from build123d import *

# Parameters (mm, degrees)
F1_DEPTH = 50.8
F2_W     = 25.4
F2_H     = 15.875
F3_DEPTH = 19.05


with BuildPart() as f1:
    # F0 (on Right) → F1 (new body)
    with BuildSketch(Plane.YZ):
        with BuildLine():
            Line((0, 0), (0, 38.1))
            Line((0, 38.1), (-6.35, 38.1))
            ThreePointArc((-6.35, 38.1), (-10.069744, 16.419744), (-31.75, 12.7))
            Line((-31.75, 12.7), (-31.75, 0))
            Line((-31.75, 0), (0, 0))
        make_face()
    extrude(amount=F1_DEPTH)

    # F2 (on face) → F3 (cut)
    with BuildSketch(Plane.XY.offset(38.1)):
        with Locations((25.4, -7.9375)):
            Rectangle(F2_W, F2_H)
    extrude(amount=-F3_DEPTH, mode=Mode.SUBTRACT)


solid = f1.part
Verification items for the finished model (mm, model axes). A direction names the side the tool comes from. Give positions to 0.01 mm unless a question says otherwise; leave off trailing zeros. Write each loop counter-clockwise with the first axis right and the second up, starting at its lowest first coordinate (ties: lowest second). Pieces come first, ordered by that corner, then holes. Notation, with made-up numbers: (-17, 69) - (5, 69) arc R24 ccw to (5, 108) - close; hole circle Ø8 at (83.25, -12). An arc over 180 degrees is marked (long way). Answer as CSV lines item,"result". Start each with the question number.
1. Sectioned sample at B-B (x = 6). Record the boundary of the cut face in (y, z), then the cut area to 3 significant figures.
2. Draft check along X on faces 3 (the face through (12.7, -3, 29)), 4 (the face through (44, -3, 38.1)), 5 (the face through (50.8, -13, 11)), 6 (the face through (0, -13, 11)). Enter one of: pulls with the +X half, pulls with the -X half, needs draft (parallel to the pull), parting line crosses it, or undercut.
3. Sectioned sample at D-D (z = 22). Record the boundary of the cut face in (x, y).
4. Depth check by flat-ended pin: pin 1 (4 mm diameter, centred on x = 7, z = 20, fed in from -Y); pin 2 (12 mm diameter, centred on x = 33.5, y = -25, fed in from +Z); pin 3 (12 mm diameter, centred on y = -26, z = 23, fed in from -X); pin 4 (2.5 mm diameter, centred on x = 26.5, y = -5.5, fed in from +Z). Enter the tip coordinate at first touch or a pass-through.
5. Thickness scan on line 1 (X direction, y = -1.5, z = 20.5); line 2 (Z direction, x = 20.5, y = -7.5); line 3 (Z direction, x = 24, y = -24). Record the ranges inside material, lowest first.
6. Sectioned sample at A-A (z = 35.5). Record the boundary of the cut face in (x, y), then the cut area to 3 significant figures.
7. Sectioned sample at C-C (y = -5.5). Record the boundary of the cut face in (x, z).
8. Set-up check for faces 1 (the face through (38.1, -3, 29)), 2 (the face through (25, -31.75, 6)): record each of +Z, -Z, +X, -X, +Y, -Y from which the full face is reachable in a straight line by a thin tool's end or side.
Derived:
1,outline,"(-31.75, 0) - (0, 0) - (0, 38.1) - (-6.35, 38.1) arc R19.05 cw to (-31.75, 12.7) - close"
1,area,"554 mm²"
2,face 3,"undercut"
2,face 4,"needs draft"
2,face 5,"pulls with the +X half"
2,face 6,"pulls with the -X half"
3,outline,"(0, -6.2) - (12.7, -6.2) - (12.7, 0) - (0, 0) - close; (38.1, -6.2) - (50.8, -6.2) - (50.8, 0) - (38.1, 0) - close"
4,pin 1,"y = -8.66"
4,pin 2,"z = 12.36"
4,pin 3,"through"
4,pin 4,"z = 19.05"
5,line 1,"0 to 12.7, 38.1 to 50.8"
5,line 2,"0 to 19.05"
5,line 3,"0 to 10.85"
6,outline,"(0, -5.33) - (12.7, -5.33) - (12.7, 0) - (0, 0) - close; (38.1, -5.33) - (50.8, -5.33) - (50.8, 0) - (38.1, 0) - close"
6,area,"136 mm²"
7,outline,"(0, 0) - (50.8, 0) - (50.8, 23.77) - (38.1, 23.77) - (38.1, 19.05) - (12.7, 19.05) - (12.7, 23.77) - (0, 23.77) - close; (0, 36.01) - (12.7, 36.01) - (12.7, 38.1) - (0, 38.1) - close; (38.1, 36.01) - (50.8, 36.01) - (50.8, 38.1) - (38.1, 38.1) - close"
8,face 1,"+Z, +Y, -Y"
8,face 2,"+Z, -Z, +X, -X, -Y"
